Could you check a few things on this model? Use its own coordinates, in mm. A direction names the side the tool comes from. Coordinates: 2 decimals unless noted, no trailing zeros. Loops run counter-clockwise (first coordinate to the right, second up) from the corner with the lowest first, then second, coordinate; pieces in that order, holes last.
Solid Edge part; units mm, degrees
sketch "Sketch1" plane through (0, 0, 0) normal (0, 0, 1) x (1, 0, 0)
  line L0 (94.5072, -47.022) -> (-94.5072, -47.022)
  line L1 (-94.5072, -47.022) -> (-94.5072, 47.022)
  line L2 (-94.5072, 47.022) -> (94.5072, 47.022)
  line L3 (94.5072, 47.022) -> (94.5072, -47.022)
extrude "Protrusion1" add sketch "Sketch1" along normal blind 42.8556
sketch "Sketch2" plane through (0, 0, 42.8556) normal (0, 0, 1) x (0, 1, 0)
  line L0 (-12.3474, 81.3483) -> (-12.3474, 28.1728)
  line L1 (-12.3474, 28.1728) -> (-33.3033, 28.1728)
  line L2 (-33.3033, 28.1728) -> (-33.3033, 81.3483)
  line L3 (-33.3033, 81.3483) -> (-12.3474, 81.3483)
extrude "ExtrudedCutout_1" cut sketch "Sketch2" against normal blind 21.544
sketch "Sketch3" plane through (0, 0, 42.8556) normal (0, 0, 1) x (0, 1, 0)
  circle A0 centre (19.417, 16.3489) radius 11
  circle A1 centre (19.417, -11) radius 11
  circle A2 centre (19.417, -38.859) radius 11
  circle A3 centre (19.417, -66.2963) radius 11
extrude "ExtrudedCutout_2" cut sketch "Sketch3" against normal blind 103.4341
sketch "Sketch4" plane through (0, 0, 0) normal (0, 0, -1) x (0, -1, 0)
  line L0 (12.4915, 83.4201) -> (35.4423, 83.4201)
  line L1 (35.4423, 83.4201) -> (35.4423, 27.3756)
  line L2 (35.4423, 27.3756) -> (12.4915, 27.3756)
  line L3 (12.4915, 27.3756) -> (12.4915, 83.4201)
  circle A0 centre (-19.417, 16.3489) radius 12.7054
  circle A1 centre (-19.417, -11) radius 12.9901
  circle A2 centre (-19.417, -38.859) radius 12.4728
  circle A3 centre (-19.417, -66.2963) radius 12.6976
  line L4 (-37.1683, 93.0942) -> (37.1336, 93.0942)
  arc A4 (37.1336, 93.0942) -> (45.7291, 84.4987) centre (37.1336, 84.4987) cw
  line L5 (45.7291, 84.4987) -> (45.7291, -84.529)
  arc A5 (45.7291, -84.529) -> (36.9537, -93.3044) centre (36.9537, -84.529) cw
  line L6 (36.9537, -93.3044) -> (-35.9897, -93.3044)
  arc A6 (-35.9897, -93.3044) -> (-45.711, -84.5471) centre (-35.9897, -83.53) cw
  line L7 (-45.711, -84.5471) -> (-45.711, 84.5189)
  arc A7 (-45.711, 84.5189) -> (-37.1683, 93.0942) centre (-37.1357, 84.5189) cw
extrude "Cutout_3" cut sketch "Sketch4" against normal blind 37.32
sketch "Sketch5" plane through (-55.3979, -12.4915, 18.6615) normal (0, 1, 0) x (-1, 0, 0)
  line L0 (-27.2251, 18.6585) -> (25.9504, 18.6585)
  line L1 (25.9504, 18.6585) -> (25.9504, 2.6501)
  line L2 (25.9504, 2.6501) -> (-27.2251, 2.6501)
  line L3 (-27.2251, 2.6501) -> (-27.2251, 18.6585)
extrude "ExtrudedProtrusion_2" add sketch "Sketch5" against normal blind 0.0041
sketch "Sketch6" plane through (-54.7605, -12.3474, 40.0894) normal (0, -1, 0) x (-1, 0, 0)
  line L0 (-26.5878, -2.7663) -> (26.5878, -2.7663)
  line L1 (26.5878, -2.7663) -> (26.5878, 18.7777)
  line L2 (26.5878, 18.7777) -> (-26.5878, 18.7777)
  line L3 (-26.5878, 18.7777) -> (-26.5878, -2.7663)
extrude "ExtrudedProtrusion_3" add sketch "Sketch6" along normal blind 0.35
draft "Draft_7" angle 8 neutral plane through (0, 0, 42.8556) normal (0, 0, 1) pull direction (0, 0, 1) face at (94.5072, 32.2884, 35.2844) face at (-64.8949, 47.022, 35.2844) face at (-94.5072, -32.2884, 35.2844) face at (64.8949, -47.022, 35.2844)
fillet "Round_1" radius 8 8 edges at (-97.5187, 50.0335, 21.4278) (-94.5072, 0, 42.8556) (0, 47.022, 42.8556) (-97.5187, -50.0335, 21.4278) (0, -47.022, 42.8556) (97.5187, -50.0335, 21.4278) (94.5072, 0, 42.8556) (97.5187, 50.0335, 21.4278)
(1) For pin 1 (3 mm diameter, centred on y = 31.5, z = 24.5, fed in from +X); pin 2 (10.5 mm diameter, centred on x = -43.5, y = -22.5, fed in from +Z); pin 3 (13 mm diameter, centred on x = 66.3, y = 19.42, fed in from +Z); pin 4 (8 mm diameter, centred on x = -50, z = 28, fed in from +Y), each with a flat end and sliding along its axis, tell me the tip position at first contact or that it passes through.
Answers:
pin 1: stops at x = 97.3
pin 2: stops at z = 21.31
pin 3: passes through
pin 4: stops at y = 49.67
(2) Imagine slicing it at A-A, the plane x = 11. Write out the boundary of the cut face in (y, z), and give its area (3 significant figures).
Answers:
outline: (-53.04, 0) - (-45.73, 0) - (-45.73, 37.32) - (6.43, 37.32) - (6.43, 0) - (8.42, 0) - (8.42, 42.86) - (-40.07, 42.86) arc R8 ccw to (-47.99, 35.97) - close; (30.42, 0) - (32.41, 0) - (32.41, 37.32) - (45.71, 37.32) - (45.71, 0) - (53.04, 0) - (47.99, 35.97) arc R8 ccw to (40.07, 42.86) - (30.42, 42.86) - close
area: 883 mm2
(3) We'd pull the mould along Y, two halves only. Please class faces 1 (the face through (22, 22, 0)), 2 (the face through (-81.348, -23, 32)), 3 (the face through (-1.297, 50.553, 17.733)): +Y half, -Y half, draft (parallel to the pull), parting line (faces both ways), or undercut.
Answers:
face 1: draft
face 2: undercut
face 3: +Y half
(4) I need wall thicknesses on probe 1 along Y at (x, z) = (-42, 36); probe 2 along Y at (x, z) = (46.5, 24); probe 3 along X at (y, z) = (-18, 9). Which ranges of each line are inside material? Lowest first, please.
Answers:
probe 1: y = -47.99 to -45.73, -35.44 to -33.3, -12.7 to -12.35, 45.71 to 47.99
probe 2: y = -49.67 to -45.73, 9.56 to 11.5, 27.33 to 29.28, 45.71 to 49.67
probe 3: x = -99.27 to -93.09, -83.42 to -27.38, 93.3 to 99.27
(5) Imagine slicing it at C-C, the plane y = -7. Write out the boundary of the cut face in (x, z).
Answers:
outline: (-100.53, 0) - (-93.09, 0) - (-93.09, 37.32) - (93.3, 37.32) - (93.3, 0) - (100.53, 0) - (95.48, 35.97) arc R8 ccw to (87.55, 42.86) - (-87.55, 42.86) arc R8 ccw to (-95.48, 35.97) - close
(6) Which directions (+Z, -Z, +X, -X, +Y, -Y) give clear straight access to the entire face, cutting with the end or side of a thin tool? Please do faces 4 (the face through (8, 47, 0)), 5 (the face through (-83.42, -24, 18)), 6 (the face through (-28.173, -23, 32)).
Answers:
face 4: -Z, +X, -X, +Y, -Y
face 5: -Z
face 6: +Z
(7) Imagine slicing it at B-B, the plane z = 13. State how many separate pieces and enclosed holes the cut face has, and give its area (3 significant figures).
Answers:
separate pieces: 6
enclosed holes: 5
area: 4,990 mm2
(8) Imagine slicing it at D-D, the plane x = -31. Write out the boundary of the cut face in (y, z), and give its area (3 significant figures).
Answers:
outline: (-53.04, 0) - (-45.73, 0) - (-45.73, 37.32) - (-35.44, 37.32) - (-35.44, 0) - (-12.49, 0) - (-12.49, 21.31) - (-12.35, 21.31) - (-12.35, 37.32) - (45.71, 37.32) - (45.71, 0) - (53.04, 0) - (47.99, 35.97) arc R8 ccw to (40.07, 42.86) - (-12.7, 42.86) - (-12.7, 21.31) - (-33.3, 21.31) - (-33.3, 42.86) - (-40.07, 42.86) arc R8 ccw to (-47.99, 35.97) - close
area: 1,270 mm2
